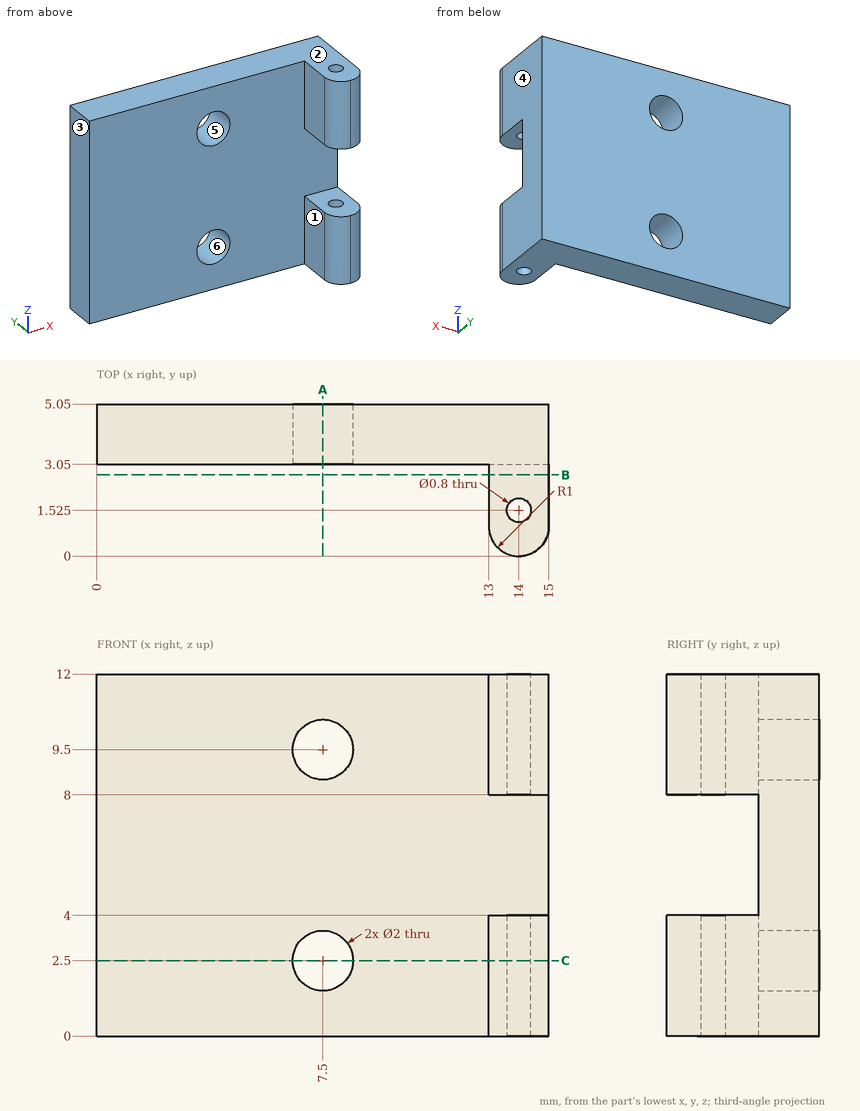
Could you check a few things on this drawing? It's one solid part, dimensions in mm from its lowest x, y, z. A direction names the side the tool comes from. Give positions to 0.01 mm unless a question says otherwise; leave off trailing zeros. Write each loop counter-clockwise with the first axis right and the second up, starting at its lowest first coordinate (ties: lowest second). Pieces come first, ordered by that corner, then holes. Notation, with made-up numbers: M 21,64.5 L 26,64.5 A15 cw 26,72.5 Z; hole C -6.75,-35.5 d8. An arc over 180 degrees is marked long. Put each result on its own line as item: value. Start each with the question number.
Item 1: On a 3-axis mill with a long thin cutter (end or side, diameter ignored), from which of +Z, -Z, +X, -X, +Y, -Y can I reach the whole of each face in a straight line? I mean the marked faces 1 and 2. Say none if no direction works.
Item 2: Will these pins go through, and if not, where does the flat tip stop? pin 1 (1 mm diameter, centred on y = 2, z = 1.5, fed in from -X); pin 2 (1.6 mm diameter, centred on x = 7.5, z = 9.5, fed in from +Y); pin 3 (2 mm diameter, centred on x = 7.5, z = 5, fed in from -Y).
Item 3: If we section it at C-C, the plane z = 2.5: Count the separate pieces of the cut face and the enclosed holes in it, then the cut area to 3 significant figures.
Item 4: If we section it at A-A, the plane x = 7.5: Write out the boundary of the cut face in (y, z).
Item 5: Thinking about a two-plate mould opening in X: for the marked faces 3, 4, 5 and 6, which applies, +X half, -X half, draft (parallel to the pull), parting line (faces both ways), or undercut?
Item 6: I need wall thicknesses on L1, parallel to Z at x = 7.5, y = 4.6; L2, parallel to Y at x = 14, z = 9.25 (3 decimals); L3, parallel to X at y = 2.7, z = 0.75. Which ranges of each line are inside material? Lowest first, please. Write a range as from..to.
Item 7: If we section it at B-B, the plane y = 2.7: Write out the boundary of the cut face in (x, z), then the cut area to 3 significant figures.
Values:
1. face 1: +Z, -Z, -X, -Y
1. face 2: +Z, +X, -X, +Y, -Y
2. pin 1: x = 13
2. pin 2: through
2. pin 3: y = 3.05
3. separate pieces: 2
3. enclosed holes: 1
3. area: 31.2 mm²
4. outline: M 3.05,0 L 5.05,0 L 5.05,1.5 L 3.05,1.5 Z; M 3.05,3.5 L 5.05,3.5 L 5.05,8.5 L 3.05,8.5 Z; M 3.05,10.5 L 5.05,10.5 L 5.05,12 L 3.05,12 Z
5. face 3: -X half
5. face 4: +X half
5. face 5: undercut
5. face 6: undercut
6. L1: 0..1.5, 3.5..8.5, 10.5..12
6. L2: 0..1.125, 1.925..5.05
6. L3: 13..15
7. outline: M 13,0 L 15,0 L 15,4 L 13,4 Z; M 13,8 L 15,8 L 15,12 L 13,12 Z
7. area: 16.0 mm²
